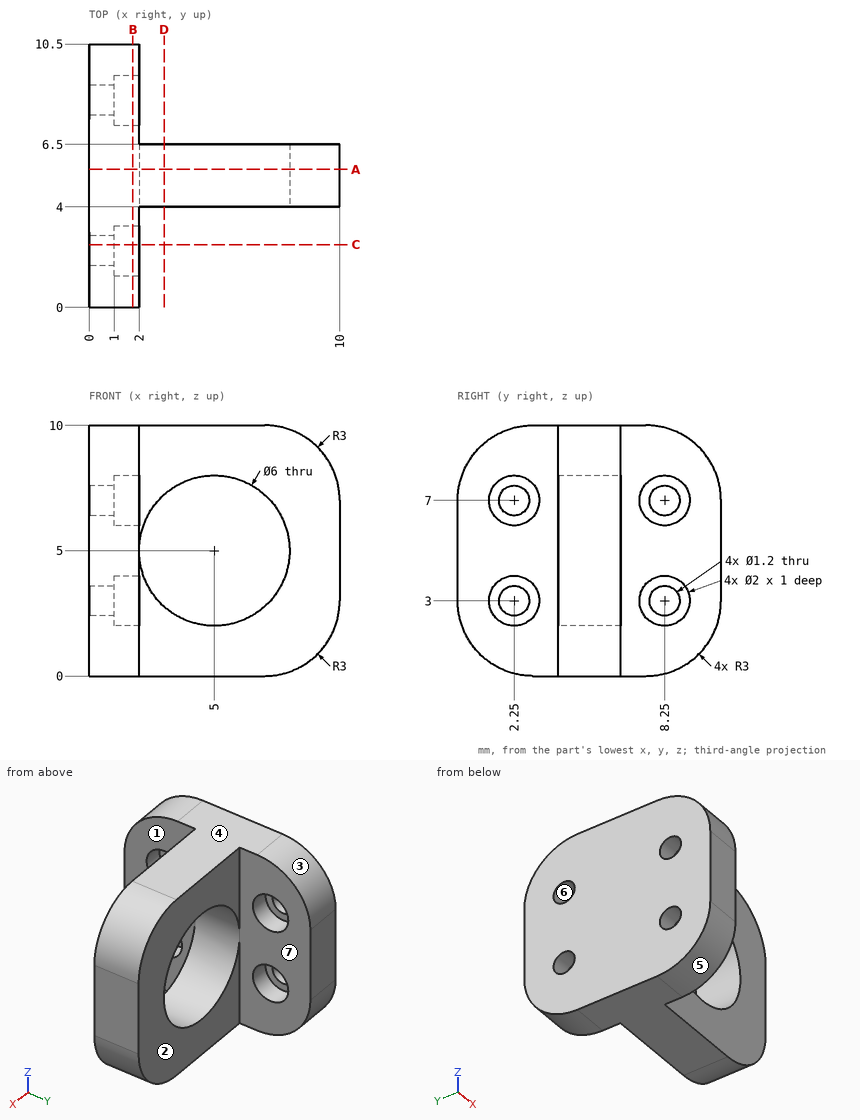
The figure shows three views and two pictorial views of one solid part (mm, origin at its lowest corner). Answer the questions. A direction names the side the tool comes from. Round coordinates to 2 decimals unless told otherwise and drop trailing zeros. Loops run counter-clockwise (first coordinate to the right, second up) from the corner with the lowest first, then second, coordinate; pieces in that order, holes last. Notation, with made-up numbers: (80.25, 71) -> (118.25, 71) arc R17 cw to (118.25, 98) -> close; hole circle Ø1 at (73, 45.5). An arc over 180 degrees is marked (long way). Use one line per item in the form item = value.
(1) Straight lines are drawn through the part: line 1 (Y direction, x = 0.5, z = 7); line 2 (Y direction, x = 1.55, z = 7); line 3 (X direction, y = 6.25, z = 3.5). For each, find the intervals that lie inside material, in ascending order.
Answer list:
line_1 = 0 to 1.65, 2.85 to 7.65, 8.85 to 10.5
line_2 = 0 to 1.25, 3.25 to 7.25, 9.25 to 10.5
line_3 = 0 to 2.4, 7.6 to 10
(2) Find section B-B on x = 1.75. Give the vertices of the cut face in (y, z), then the cut area to 3 significant figures.
Answer list:
outline = (0, 3) arc R3 ccw to (3, 0) -> (7.5, 0) arc R3 ccw to (10.5, 3) -> (10.5, 7) arc R3 ccw to (7.5, 10) -> (3, 10) arc R3 ccw to (0, 7) -> close; hole circle Ø2 at (2.25, 3); hole circle Ø2 at (2.25, 7); hole circle Ø2 at (8.25, 3); hole circle Ø2 at (8.25, 7)
area = 84.7 mm2
(3) For a pull along Z with two mould halves and no side action, classify the marked faces 4, 5, 6 and 7 as released by +Z, released by -Z, zero draft, split by the parting line, or undercut.
Answer list:
face_4 = released by +Z
face_5 = released by -Z
face_6 = undercut
face_7 = zero draft
(4) Find section A-A on y = 5.5. Give the vertices of the cut face in (x, z), then the cut area to 3 significant figures.
Answer list:
outline = (0, 0) -> (7, 0) arc R3 ccw to (10, 3) -> (10, 7) arc R3 ccw to (7, 10) -> (0, 10) -> close; hole circle Ø6 at (5, 5)
area = 67.9 mm2
(5) A tool of negligible diameter and unlimited length cuts with its end or side. For the marked faces 1, 2 and 3, from which of +Z, -Z, +X, -X, +Y, -Y can it reach the whole face along a straight path? Write none if from no direction.
Answer list:
face_1 = +Z, -Z, +X, -Y
face_2 = +Z, -Z, +X, +Y
face_3 = +Z, +X, -X, +Y
(6) Flat-ended cylindrical pins translate along their axes: P1, Ø1.6, axis at y = 8.25, z = 3, coming from the +X side; P2, Ø3, axis at x = 4.5, z = 3, coming from the +Y side; P3, Ø1.9, axis at y = 2.25, z = 3, coming from the -X side; P4, Ø0.6, axis at y = 2, z = 7, coming from the +X side. Find the tip coordinate at first contact, or state that the pin passes through.
Answer list:
P1 = 1
P2 = 6.5
P3 = 0
P4 = through
(7) Find section D-D on x = 3. Give the vertices of the cut face in (y, z), then the cut area to 3 significant figures.
Answer list:
outline = (4, 0) -> (6.5, 0) -> (6.5, 2.76) -> (4, 2.76) -> close; (4, 7.24) -> (6.5, 7.24) -> (6.5, 10) -> (4, 10) -> close
area = 13.8 mm2
(8) Find section C-C on y = 2.5. Give the vertices of the cut face in (x, z).
Answer list:
outline = (0, 0.04) -> (2, 0.04) -> (2, 2.03) -> (1, 2.03) -> (1, 2.45) -> (0, 2.45) -> close; (0, 3.55) -> (1, 3.55) -> (1, 3.97) -> (2, 3.97) -> (2, 6.03) -> (1, 6.03) -> (1, 6.45) -> (0, 6.45) -> close; (0, 7.55) -> (1, 7.55) -> (1, 7.97) -> (2, 7.97) -> (2, 9.96) -> (0, 9.96) -> close
